```python
from build123d import *

# Parameters (mm, degrees)
F2_SIZE  = 0.5
F3_R     = 5
F3_R_2   = 3.5
F4_DEPTH = 0.4
F5_R     = 2
F6_R     = 1.6
F7_DEPTH = 25
F8_R     = 3
F8_R_2   = 1.6
F9_DEPTH = 2.5


# Not quite as in the source:
# - a feature names something its author has since deleted; it is built from what else it names


with BuildPart() as f1:
    # F0 (on Front) → F1 (revolve)
    with BuildSketch(Plane.XZ):
        Polygon((3.5, 6), (0, 6), (0, 0), (10, 0), (10, 3), (3.5, 3), align=None)
    revolve(axis=Axis((0, 0, 3), (0, 0, -1)))

    # F2
    f2_edges = [f1.edges().sort_by_distance(p)[0] for p in [
        (-3.5, 0, 6),
    ]]
    chamfer(f2_edges, length=F2_SIZE)

    # F3 (on face) → F4 (join)
    with BuildSketch(Plane.XY.offset(3)):
        Circle(F3_R)
        Circle(F3_R_2, mode=Mode.SUBTRACT)
    extrude(amount=F4_DEPTH)

    # F5
    f5_edges = [f1.edges().sort_by_distance(p)[0] for p in [
        (-10, 0, 0),
    ]]
    fillet(f5_edges, radius=F5_R)

    # F6 (on face) → F7 (cut)
    with BuildSketch(Plane.XY.offset(6)):
        Circle(F6_R)
    extrude(amount=-F7_DEPTH, mode=Mode.SUBTRACT)

    # F8 (on face) → F9 (cut)
    with BuildSketch(Plane(origin=(0, 0, 0), x_dir=(1, 0, 0), z_dir=(0, 0, -1))):
        Circle(F8_R)
        Circle(F8_R_2, mode=Mode.SUBTRACT)
    extrude(amount=-F9_DEPTH, mode=Mode.SUBTRACT)


solid = f1.part
```
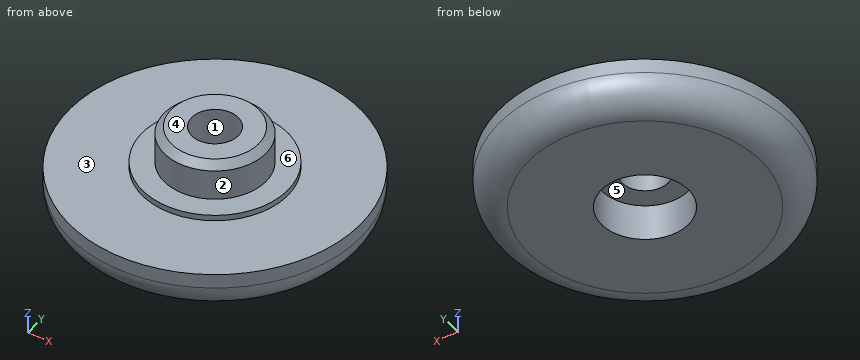
Check sheet for the modelled part. Datum: model origin and axes. Units: mm. Face numbers are marked on the shaded views. A direction names the side the tool comes from. Round coordinates to 2 decimals unless told otherwise and drop trailing zeros. Loops run counter-clockwise (first coordinate to the right, second up) from the corner with the lowest first, then second, coordinate; pieces in that order, holes last. Notation, with made-up numbers: (25.25, 68.5) - (36.25, 68.5) arc R12 cw to (36.25, 86.5) - close; hole circle Ø11 at (-23.5, -6.75). An arc over 180 degrees is marked (long way). Answer as a JSON object with one key per item and string values. Group by question number.
Q1. Sectioned sample at D-D, the plane z = 1.65. Enter the section's corners in (x, y), plus the area to 3 significant figures.
Q2. Mould release check, pull along Y, two halves, no side actions. Record for the marked faces 1, 2 and 3: released by +Y, released by -Y, zero draft, split by the parting line, or undercut.
Q3. Scan lines: line 1 along Y through (x, z) = (0, 5.25); line 2 along Y through (x, z) = (0, 3.3). Record each from-to range of solid material in increasing order. Write a range as [from, to].
Q4. Sectioned sample at C-C, the plane z = 4.9. Enter the section's corners in (x, y).
Q5. Gauge pin test, flat ends, axial feed: P1, Ø3.5, axis at x = 0, y = 0, coming from the -Z side; P2, Ø1, axis at x = 1.5, y = -5, coming from the +Z side; P3, Ø3, axis at y = -6.5, z = 2.5, coming from the +X side; P4, Ø2.5, axis at x = 0, y = 0, coming from the -Z side. Record the tip position at first contact, or that the pin passes through.
Q6. Sectioned sample at A-A, the plane x = 0. Enter the section's corners in (y, z).
Q7. Set-up check for the marked faces 4, 5 and 6: record each of +Z, -Z, +X, -X, +Y, -Y from which the full face is reachable in a straight line by a thin tool's end or side.
Solution:
{
 "1": {"outline": "circle Ø19.94 at (0, 0); hole circle Ø6 at (0, 0)", "area": "284 mm²"},
 "2": {"face 1": "undercut", "face 2": "split by the parting line", "face 3": "zero draft"},
 "3": {"line 1": "y = [-3.5, -1.6], [1.6, 3.5]", "line 2": "y = [-5, -1.6], [1.6, 5]"},
 "4": {"outline": "circle Ø7 at (0, 0); hole circle Ø3.2 at (0, 0)"},
 "5": {"P1": "stops at z = 2.5", "P2": "stops at z = 3.4", "P3": "stops at x = 8.66", "P4": "passes through"},
 "6": {"outline": "(-10, 2) arc R2 ccw to (-8, 0) - (-3, 0) - (-3, 2.5) - (-1.6, 2.5) - (-1.6, 6) - (-3, 6) - (-3.5, 5.5) - (-3.5, 3.4) - (-5, 3.4) - (-5, 3) - (-10, 3) - close; (1.6, 2.5) - (3, 2.5) - (3, 0) - (8, 0) arc R2 ccw to (10, 2) - (10, 3) - (5, 3) - (5, 3.4) - (3.5, 3.4) - (3.5, 5.5) - (3, 6) - (1.6, 6) - close"},
 "7": {"face 4": "+Z, +X, -X, +Y, -Y", "face 5": "-Z", "face 6": "+Z"}
}
